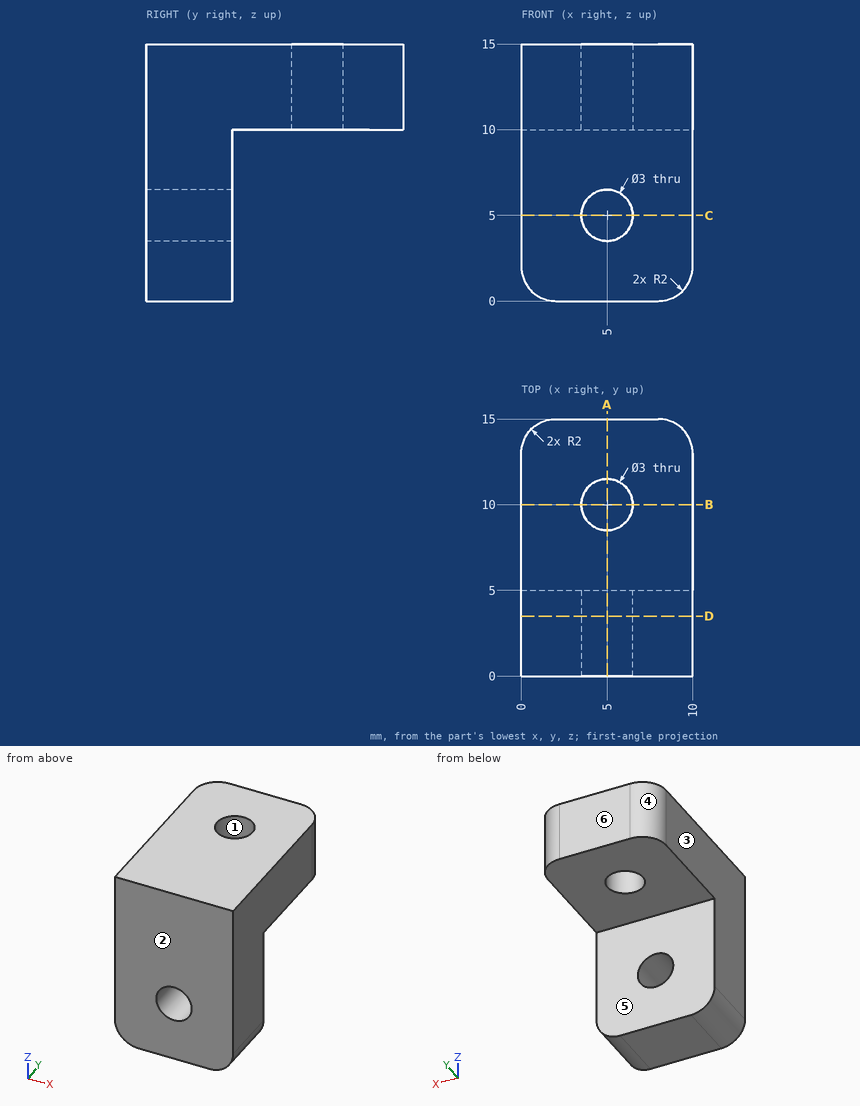
For this review, use the dimensioned drawing (mm, ordinates from the lowest corner) and the shaded views. A direction names the side the tool comes from. Round coordinates to 2 decimals unless told otherwise and drop trailing zeros. Write each loop counter-clockwise with the first axis right and the second up, starting at its lowest first coordinate (ties: lowest second). Pieces come first, ordered by that corner, then holes. Notation, with made-up numbers: (-23, 73) -> (27, 73) arc R29 cw to (27, 98) -> close; hole circle Ø5 at (23.25, 63.25). An arc over 180 degrees is marked (long way). One line per item, written item: value. Start each with the question number.
Q1. Add section D-D (y = 3.5). Give the boundary of the cut face in (x, z), then the cut area to 3 significant figures.
Q2. Add section B-B (y = 10). Give the boundary of the cut face in (x, z), then the cut area to 3 significant figures.
Q3. To check wall thickness, follow probe 1 along X at (y, z) = (10, 13.1); probe 2 along Y at (x, z) = (5, 13.1); probe 3 along Z at (x, y) = (5, 1.75). State the ranges of each line that lie inside material, in increasing order.
Q4. Add section A-A (x = 5). Give the boundary of the cut face in (y, z).
Q5. Add section C-C (z = 5). Give the boundary of the cut face in (x, y), then the cut area to 3 significant figures.
Q6. Insertion check: P1, Ø5, axis at x = 5, z = 1.5, coming from the +Y side; P2, Ø1, axis at x = 3.5, y = 10.5, coming from the -Z side. Each pin has a flat end and moves straight along its axis. Give the tip position at first contact, or say it passes through.
Q7. The part is to be moulded in two halves that separate along Y. For the marked faces 1, 2, 3 and 4, say which applies: pulls with the +Y half, pulls with the -Y half, needs draft (parallel to the pull), parting line crosses it, or undercut.
Q8. Tool access review of the marked faces 5 and 6: name each direction out of +Z, -Z, +X, -X, +Y, -Y from which nothing blocks a thin tool from reaching the whole face with its end or side.
Response:
1. outline: (0, 2) arc R2 ccw to (2, 0) -> (8, 0) arc R2 ccw to (10, 2) -> (10, 15) -> (0, 15) -> close; hole circle Ø3 at (5, 5)
1. area: 141 mm^2
2. outline: (0, 10) -> (3.5, 10) -> (3.5, 15) -> (0, 15) -> close; (6.5, 10) -> (10, 10) -> (10, 15) -> (6.5, 15) -> close
2. area: 35.0 mm^2
3. probe 1: x = 0 to 3.5, 6.5 to 10
3. probe 2: y = 0 to 8.5, 11.5 to 15
3. probe 3: z = 0 to 3.5, 6.5 to 15
4. outline: (0, 0) -> (5, 0) -> (5, 3.5) -> (0, 3.5) -> close; (0, 6.5) -> (5, 6.5) -> (5, 10) -> (8.5, 10) -> (8.5, 15) -> (0, 15) -> close; (11.5, 10) -> (15, 10) -> (15, 15) -> (11.5, 15) -> close
5. outline: (0, 0) -> (3.5, 0) -> (3.5, 5) -> (0, 5) -> close; (6.5, 0) -> (10, 0) -> (10, 5) -> (6.5, 5) -> close
5. area: 35.0 mm^2
6. P1: stops at y = 5
6. P2: stops at z = 10
7. face 1: undercut
7. face 2: pulls with the -Y half
7. face 3: needs draft
7. face 4: pulls with the +Y half
8. face 5: -Z, +X, -X, +Y
8. face 6: +Z, -Z, +X, -X, +Y
